```python
from build123d import *

# Parameters (mm, degrees)
BOSS_EXTRUDE1_DEPTH = 19.5
BOSS_EXTRUDE2_START = 18.5
SKETCH2_3_R         = 2.250000000000002
SKETCH2_3_R_2       = 2.249999999999999
BOSS_EXTRUDE2_DEPTH = 1
BOSS_EXTRUDE3_START = 19.5
SKETCH2_4_R         = 4.5
SKETCH2_4_R_2       = 2.5000000000000004
SKETCH2_4_W         = 3
SKETCH2_4_H         = 3.9999999999999973
BOSS_EXTRUDE3_DEPTH = 1
BOSS_EXTRUDE4_START = 20.5
SKETCH2_5_W         = 3
SKETCH2_5_H         = 3.9999999999999973
BOSS_EXTRUDE4_DEPTH = 2
BOSS_EXTRUDE5_START = 22.5
SKETCH2_6_W         = 3
SKETCH2_6_H         = 3.9999999999999973
BOSS_EXTRUDE5_DEPTH = 6.5


with BuildPart() as part:
    # Sketch2 → Boss-Extrude1 (new body)
    with BuildSketch(Plane(origin=(0, 0, 0), x_dir=(1, 0, 0), z_dir=(0, 1, 0))):
        with BuildLine():
            Line((-8.500000000000002, -17), (8.499999999999998, -17))
            Line((8.499999999999998, -17), (8.499999999999998, -11.124297730643494))
            ThreePointArc((8.5, -11.124297730643494), (0, 14), (-8.5, -11.124297730643493))
            Line((-8.500000000000002, -11.124297730643494), (-8.500000000000002, -17))
        make_face()
    extrude(amount=BOSS_EXTRUDE1_DEPTH)

    # Sketch2<3> → Boss-Extrude2 (add)
    # profile 1 of 2: a face of its own
    with BuildSketch(Plane(origin=(0, 0, 0), x_dir=(1, 0, 0), z_dir=(0, 1, 0)).offset(BOSS_EXTRUDE2_START)):
        with BuildLine():
            Line((13.555441711725987, -3.4999999999999996), (17.5, -3.499999999999999))
            ThreePointArc((17.5, -3.5), (21, -2.4e-16), (17.5, 3.5))
            Line((17.5, 3.499999999999999), (13.555441711725718, 3.4999999999999987))
            ThreePointArc((13.555441711725832, 3.5000000000004934), (13.999999999999998, 2.8244e-13), (13.555441711725974, -3.4999999999999454))
        make_face()
        with Locations(Location((17.5, -3e-17, 0), (0, 0, 270))):
            Circle(SKETCH2_3_R, mode=Mode.SUBTRACT)
    # profile 2 of 2: a face of its own
    with BuildSketch(Plane(origin=(0, 0, 0), x_dir=(1, 0, 0), z_dir=(0, 1, 0)).offset(BOSS_EXTRUDE2_START)):
        with BuildLine():
            Line((-17.499999999999986, -3.5000000000000044), (-13.555441711725983, -3.500000000000004))
            ThreePointArc((-13.555441711725972, -3.4999999999999547), (-14.000000000000002, 2.7667e-13), (-13.555441711725834, 3.50000000000049))
            Line((-13.55544171172572, 3.499999999999996), (-17.499999999999986, 3.4999999999999956))
            ThreePointArc((-17.499999999999986, 3.4999999999999956), (-20.999999999999986, -3.91e-15), (-17.499999999999986, -3.5000000000000044))
        make_face()
        with Locations(Location((-17.499999999999986, -4.34e-15, 0), (0, 0, 270))):
            Circle(SKETCH2_3_R_2, mode=Mode.SUBTRACT)
    extrude(amount=BOSS_EXTRUDE2_DEPTH)

    # Sketch2<4> → Boss-Extrude3 (add)
    # profile 1 of 6: a face of its own
    with BuildSketch(Plane(origin=(0, 0, 0), x_dir=(1, 0, 0), z_dir=(0, 1, 0)).offset(BOSS_EXTRUDE3_START)):
        with Locations(Location((0, 8.5, 0), (0, 0, 270))):
            Circle(SKETCH2_4_R)
        with Locations((0, 8.5)):
            Circle(SKETCH2_4_R_2, mode=Mode.SUBTRACT)
    # profile 2 of 6: a face of its own
    with BuildSketch(Plane(origin=(0, 0, 0), x_dir=(1, 0, 0), z_dir=(0, 1, 0)).offset(BOSS_EXTRUDE3_START)):
        with Locations((0, 8.5)):
            Circle(SKETCH2_4_R_2)
    # profile 3 of 6: a face of its own
    with BuildSketch(Plane(origin=(0, 0, 0), x_dir=(1, 0, 0), z_dir=(0, 1, 0)).offset(BOSS_EXTRUDE3_START)):
        with BuildLine():
            ThreePointArc((-1.5000000000000007, 10.5), (-2.5000000000000004, 8.5), (-1.5000000000000004, 6.5))
            Line((-1.5, 6.500000000000001), (-1.5, 10.499999999999998))
        make_face()
    # profile 4 of 6: a face of its own
    with BuildSketch(Plane(origin=(0, 0, 0), x_dir=(1, 0, 0), z_dir=(0, 1, 0)).offset(BOSS_EXTRUDE3_START)):
        with BuildLine():
            Line((-1.5, 10.499999999999998), (1.5, 10.499999999999998))
            ThreePointArc((1.500000000000001, 10.5), (1.5e-16, 11), (-1.5000000000000007, 10.5))
        make_face()
    # profile 5 of 6: a face of its own
    with BuildSketch(Plane(origin=(0, 0, 0), x_dir=(1, 0, 0), z_dir=(0, 1, 0)).offset(BOSS_EXTRUDE3_START)):
        with Locations((0, 8.5)):
            Rectangle(SKETCH2_4_W, SKETCH2_4_H)
    # profile 6 of 6: a face of its own
    with BuildSketch(Plane(origin=(0, 0, 0), x_dir=(1, 0, 0), z_dir=(0, 1, 0)).offset(BOSS_EXTRUDE3_START)):
        with BuildLine():
            ThreePointArc((-1.5000000000000004, 6.5), (-4.6e-16, 6), (1.4999999999999996, 6.499999999999999))
            Line((1.5, 6.500000000000001), (-1.5, 6.500000000000001))
        make_face()
    extrude(amount=BOSS_EXTRUDE3_DEPTH)

    # Sketch2<5> → Boss-Extrude4 (add)
    with BuildSketch(Plane(origin=(0, 0, 0), x_dir=(1, 0, 0), z_dir=(0, 1, 0)).offset(BOSS_EXTRUDE4_START)):
        with BuildLine():
            ThreePointArc((-1.5000000000000004, 6.5), (-4.6e-16, 6), (1.4999999999999996, 6.499999999999999))
            Line((1.5, 6.500000000000001), (-1.5, 6.500000000000001))
        make_face()
        with Locations((0, 8.5)):
            Rectangle(SKETCH2_5_W, SKETCH2_5_H)
        with BuildLine():
            Line((1.5, 10.499999999999998), (1.5, 6.500000000000001))
            ThreePointArc((1.4999999999999996, 6.499999999999999), (2.23606797749979, 7.381966011250104), (2.5000000000000004, 8.5))
            ThreePointArc((2.5000000000000004, 8.5), (2.2360679774997902, 9.618033988749895), (1.5000000000000013, 10.5))
        make_face()
        with BuildLine():
            ThreePointArc((-1.5000000000000007, 10.5), (-2.5000000000000004, 8.5), (-1.5000000000000004, 6.5))
            Line((-1.5, 6.500000000000001), (-1.5, 10.499999999999998))
        make_face()
        with BuildLine():
            Line((-1.5, 10.499999999999998), (1.5, 10.499999999999998))
            ThreePointArc((1.500000000000001, 10.5), (1.5e-16, 11), (-1.5000000000000007, 10.5))
        make_face()
    extrude(amount=BOSS_EXTRUDE4_DEPTH)

    # Sketch2<6> → Boss-Extrude5 (add)
    with BuildSketch(Plane(origin=(0, 0, 0), x_dir=(1, 0, 0), z_dir=(0, 1, 0)).offset(BOSS_EXTRUDE5_START)):
        with BuildLine():
            ThreePointArc((-1.5000000000000004, 6.5), (-4.6e-16, 6), (1.4999999999999996, 6.499999999999999))
            Line((1.5, 6.500000000000001), (-1.5, 6.500000000000001))
        make_face()
        with Locations((0, 8.5)):
            Rectangle(SKETCH2_6_W, SKETCH2_6_H)
        with BuildLine():
            Line((-1.5, 10.499999999999998), (1.5, 10.499999999999998))
            ThreePointArc((1.500000000000001, 10.5), (1.5e-16, 11), (-1.5000000000000007, 10.5))
        make_face()
    extrude(amount=BOSS_EXTRUDE5_DEPTH)


solid = part.part
```
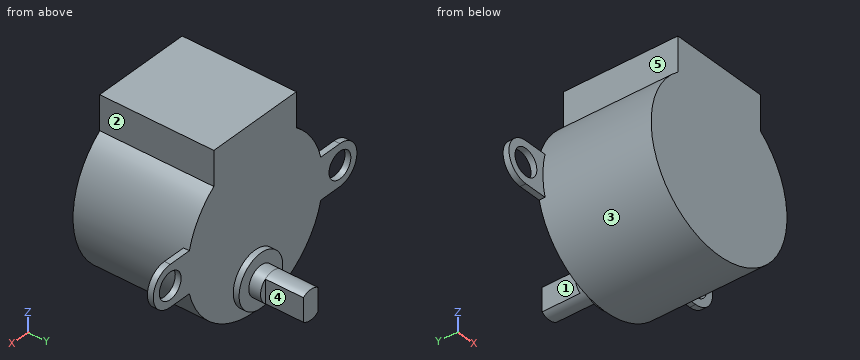
Verification items for the finished model (mm, model axes). Face numbers are marked on the shaded views. A direction names the side the tool comes from. Round coordinates to 2 decimals unless told otherwise and drop trailing zeros. Write each loop counter-clockwise with the first axis right and the second up, starting at its lowest first coordinate (ties: lowest second). Pieces come first, ordered by that corner, then holes. Notation, with made-up numbers: (57, -18) - (61, -18) arc R12 ccw to (61, -3) - close; hole circle Ø11 at (41.25, 19). An arc over 180 degrees is marked (long way). Answer as a JSON object with one key per item and string values. Group by question number.
Q1. Go/stop test with flat-tipped pins: pin 1 Ø0.8 at (x, y) = (-15.5, 19) entering from +Z; pin 2 Ø4.5 at (y, z) = (11, 14.5) entering from -X; pin 3 Ø1.2 at (y, z) = (26.5, -9.5) entering from +X. Record where each tip stops, or that it passes through.
Q2. Tool access check on the marked faces 1, 2, 3, 4 and 5. Record the directions out of +Z, -Z, +X, -X, +Y, -Y that give a thin tool (end or side, any length) a straight path to the whole face; none if there is none.
Q3. Thickness scan on line 1 (X direction, y = 18.9, z = 0); line 2 (Y direction, x = 2, z = -13); line 3 (X direction, y = 26.25, z = -7.5). Record the ranges inside material, lowest first.
Q4. Section check A-A, the plane z = 0. Enter the section's corners in (x, y), plus the area to 3 significant figures.
Q5. Section check B-B, the plane x = 0. Enter the section's corners in (y, z).
Q6. Section check C-C, the plane x = 16. Enter the section's corners in (y, z), plus the area to 3 significant figures.
Q7. Section check D-D, the plane z = -8.5. Enter the section's corners in (x, y), plus the area to 3 significant figures.
Found:
{
 "1": {"pin 1": "stops at z = 3.5", "pin 2": "stops at x = -8.5", "pin 3": "stops at x = 1.5"},
 "2": {"face 1": "+Z, -Z, -X, +Y", "face 2": "+Z, +X, +Y, -Y", "face 3": "-Y", "face 4": "+Z, -Z, +X, +Y", "face 5": "+Z, -X, +Y, -Y"},
 "3": {"line 1": "x = -21 to -19.75, -15.25 to 15.25, 19.75 to 21", "line 2": "y = 0 to 19.5", "line 3": "x = -1.5 to 1.5"},
 "4": {"outline": "(-21, 18.5) - (-19.75, 18.5) - (-19.75, 19.5) - (-21, 19.5) - close; (-15.25, 18.5) - (-14, 18.5) - (-14, 0) - (14, 0) - (14, 18.5) - (15.25, 18.5) - (15.25, 19.5) - (-15.25, 19.5) - close; (19.75, 18.5) - (21, 18.5) - (21, 19.5) - (19.75, 19.5) - close", "area": "551 mm^2"},
 "5": {"outline": "(0, -14) - (19.5, -14) - (19.5, -13) - (20.5, -13) - (20.5, -11) - (29, -11) - (29, -6) - (20.5, -6) - (20.5, -4) - (19.5, -4) - (19.5, 17) - (0, 17) - close"},
 "6": {"outline": "(18.5, -3.5) - (19.5, -3.5) - (19.5, -1.68) - (18.5, -1.68) - close; (18.5, 1.68) - (19.5, 1.68) - (19.5, 3.5) - (18.5, 3.5) - close", "area": "3.65 mm^2"},
 "7": {"outline": "(-11.12, 0) - (11.12, 0) - (11.12, 19.5) - (4.5, 19.5) - (4.5, 20.5) - (2.5, 20.5) - (2.5, 22.5) - (1.5, 22.5) - (1.5, 29) - (-1.5, 29) - (-1.5, 22.5) - (-2.5, 22.5) - (-2.5, 20.5) - (-4.5, 20.5) - (-4.5, 19.5) - (-11.12, 19.5) - close", "area": "472 mm^2"}
}
